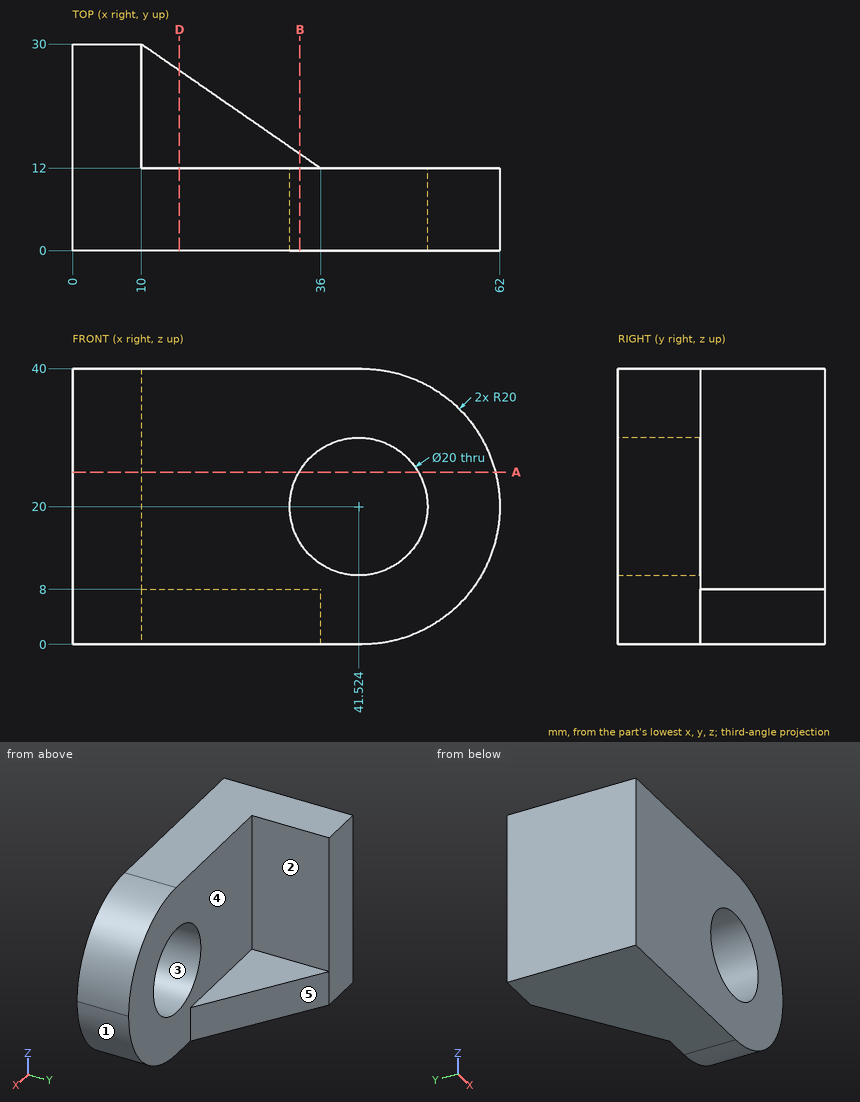
The figure shows three views and two pictorial views of one solid part (mm, origin at its lowest corner). Answer the questions. A direction names the side the tool comes from. Give positions to 0.01 mm unless a question says otherwise; leave off trailing zeros. Write each loop counter-clockwise with the first axis right and the second up, starting at its lowest first coordinate (ties: lowest second). Pieces come first, ordered by that corner, then holes.
Q1. The part is cut by section D-D on x = 15.5. Give the vertices of the cut face in (y, z).
Answer:
outline: (0, 0) - (26.19, 0) - (26.19, 8) - (12, 8) - (12, 40) - (0, 40) - close
Q2. The part is cut by section A-A on z = 25. Give the vertices of the cut face in (x, y) (1 decimal).
Answer:
outline: (0, 0) - (32.9, 0) - (32.9, 12) - (10, 12) - (10, 30) - (0, 30) - close; (50.2, 0) - (61.4, 0) - (61.4, 12) - (50.2, 12) - close
Q3. The part is cut by section B-B on x = 33. Give the vertices of the cut face in (y, z), and give its area (3 significant figures).
Answer:
outline: (0, 0) - (14.08, 0) - (14.08, 8) - (12, 8) - (12, 14.77) - (0, 14.77) - close; (0, 25.23) - (12, 25.23) - (12, 40) - (0, 40) - close
area: 371 mm2
Q4. Given pin 1 (9 mm diameter, centred on y = 23.5, z = 19.5, fed in from +X); pin 2 (9 mm diameter, centred on x = 18, y = 18, fed in from +Z); pin 3 (20 mm diameter, centred on x = 45.5, z = 24, fed in from +Y), each flat-ended and moving along its own axis, determine where each tip first touches the part or whether it passes through.
Answer:
pin 1: stops at x = 10
pin 2: stops at z = 8
pin 3: stops at y = 12
Q5. For a pull along Z with two mould halves and no side action, classify the marked faces 1, 2 and 3 as released by +Z, released by -Z, zero draft, split by the parting line, or undercut.
Answer:
face 1: released by -Z
face 2: zero draft
face 3: undercut
Q6. Straight lines are drawn through the part: L1, parallel to X at y = 5, z = 20; L2, parallel to Z at x = 42, y = 10.25; L3, parallel to X at y = 24.75, z = 20. For each, find the intervals that lie inside material, in ascending order.
Answer:
L1: x = 0 to 31.52, 51.52 to 62
L2: z = 0 to 10.01, 29.99 to 40
L3: x = 0 to 10
Q7. A tool of negligible diameter and unlimited length cuts with its end or side. For the marked faces 4 and 5, from which of +Z, -Z, +X, -X, +Y, -Y can it reach the whole face along a straight path? Write none if from no direction.
Answer:
face 4: +Z, +X, +Y
face 5: +Z, -Z, +X, +Y
